from build123d import *

# Parameters (mm, degrees)
BOSS_EXTRUDE2_DEPTH = 6.35
CUT_EXTRUDE1_DEPTH  = 7.3500001
BOSS_EXTRUDE3_DEPTH = 6.35
SKETCH10_R          = 3.96875
CUT_EXTRUDE2_DEPTH  = 7.35
SKETCH11_R          = 4.5
CUT_EXTRUDE4_DEPTH  = 7.35
BOSS_EXTRUDE4_DEPTH = 6.35
SKETCH13_R          = 3.96875
CUT_EXTRUDE5_DEPTH  = 7.35
LPATTERN1_COUNT     = 2
LPATTERN1_PITCH     = 64
SKETCH14_R          = 2.54
CUT_EXTRUDE6_DEPTH  = 7.35
SKETCH15_R          = 3.96875
CUT_EXTRUDE7_DEPTH  = 7.35
SKETCH16_R          = 3.96875
CUT_EXTRUDE8_DEPTH  = 7.35
SKETCH19_R          = 3.96875
CUT_EXTRUDE11_DEPTH = 7.35
SKETCH21_R          = 2.54
CUT_EXTRUDE12_DEPTH = 7.35
SKETCH22_R          = 31.75
CUT_EXTRUDE13_DEPTH = 7.35
SKETCH23_R          = 5.807663874
SKETCH23_R_2        = 5.610358505
BOSS_EXTRUDE5_DEPTH = 6.35
SKETCH24_R          = 10.761293976
SKETCH24_R_2        = 16.881729782
SKETCH24_R_3        = 7.918988805
BOSS_EXTRUDE6_DEPTH = 6.35
CUT_EXTRUDE14_DEPTH = 7.35
FILLET1_R           = 3.175


with BuildPart() as part:
    # Sketch6 → Boss-Extrude2 (new body)
    with BuildSketch(Plane.XY):
        with BuildLine():
            Line((-68.006850091, -76.67090114), (-109.486767671, -48.656527855))
            Line((-109.486767671, -48.656527855), (-118.371760678, -61.812230963))
            Line((-118.371760678, -61.812230963), (18.447551645, -154.216158235))
            Line((18.447551645, -154.216158235), (135.729459338, 19.43912279))
            Line((135.729459338, 19.43912279), (-1.089852986, 111.843050063))
            Line((-1.089852986, 111.843050063), (-73.946795643, 3.966284577))
            Line((-73.946795643, 3.966284577), (-56.624438948, -7.732749433))
            ThreePointArc((-56.624438948, -7.732749433), (-43.058385537, 37.577891571), (0, 57.15))
            ThreePointArc((0, 57.15), (56.404848571, 31.095576642), (70.829334649, -29.338471048))
            add(Edge.make_bspline(
                [(70.829334649, -29.338471048), (70.811686062, -29.418295928), (70.776015112, -29.578104383), (70.713320217, -29.85478305), (70.619021771, -30.262929245), (70.501052001, -30.762086912), (70.364034474, -31.322191481), (70.199318515, -31.970958926), (70.000453855, -32.723919765), (69.795103485, -33.469783355), (69.582015398, -34.214296028), (69.361377803, -34.956693289), (69.133257682, -35.696762218), (68.838782679, -36.61892651), (68.470566207, -37.720710028), (68.019498024, -38.998776477), (67.474836154, -40.448808619), (66.901337925, -41.887676852), (66.299328392, -43.31485223), (65.669141732, -44.729810424), (65.011119088, -46.132040323), (64.325609411, -47.52103904), (63.612968547, -48.896314904), (62.87355937, -50.257385735), (62.107751613, -51.603779381), (61.315921169, -52.935034173), (60.49845004, -54.250698756), (59.655726138, -55.550331897), (58.571247582, -57.154294757), (57.220953058, -59.045283389), (55.576035723, -61.200397094), (53.604026134, -63.590264702), (51.54329346, -65.904053004), (49.39728314, -68.138962994), (47.169496434, -70.29235602), (44.863486103, -72.361752995), (42.482847363, -74.344831806), (40.031215607, -76.239428526), (36.882516177, -78.494556171), (32.976808929, -81.016011003), (28.250788286, -83.68089187), (21.41551215, -86.919136497), (14.30829026, -89.526654921), (6.996956895, -91.488176442), (-0.451922312, -92.797413176), (-6.61686174, -93.456358442), (-12.81195397, -93.702029749), (-19.009644204, -93.537285056), (-25.183124422, -92.966685286), (-31.306438312, -91.996382122), (-36.598524037, -90.804323442), (-41.072542301, -89.543185606), (-44.752319298, -88.33589156), (-47.664184976, -87.27761875), (-50.541347258, -86.128353728), (-53.381128552, -84.889612663), (-56.180924218, -83.562977818), (-58.593536599, -82.326710176), (-60.633378351, -81.214215821), (-62.313751085, -80.252471782), (-63.646071553, -79.462491566), (-64.966093336, -78.652178853), (-66.222359154, -77.854259082), (-67.143044791, -77.250601571), (-67.736251212, -76.85365602), (-68.006850091, -76.67090114)],
                knots=[0.071020771, 0.071020771, 0.071020771, 0.071020771, 0.071020771, 0.072848477, 0.074676184, 0.07650389, 0.078331597, 0.08198701, 0.085642423, 0.089297836, 0.092953249, 0.096608662, 0.100264075, 0.103919488, 0.107574901, 0.114885727, 0.122196554, 0.12950738, 0.136818214, 0.144129048, 0.151439882, 0.158750716, 0.166061558, 0.173372401, 0.180683243, 0.187994085, 0.195304924, 0.202615763, 0.209926602, 0.217237441, 0.231859103, 0.246480766, 0.261102426, 0.275724085, 0.290345754, 0.304967424, 0.319589099, 0.334210774, 0.348832457, 0.36345414, 0.392697464, 0.421940789, 0.451184112, 0.506140643, 0.535383973, 0.564627303, 0.593870641, 0.623113979, 0.652357319, 0.68160066, 0.710843985, 0.740087309, 0.754708984, 0.769330659, 0.783952333, 0.798574008, 0.813195669, 0.82781733, 0.842438991, 0.849749821, 0.857060652, 0.86437149, 0.871682327, 0.878993165, 0.885158103, 0.885158103, 0.885158103, 0.885158103, 0.885158103], degree=4))
        make_face()
    extrude(amount=BOSS_EXTRUDE2_DEPTH)

    # Sketch8 → Cut-Extrude1 (cut, through all)
    with BuildSketch(Plane.XY.offset(6.35)):
        Polygon((-71.011229489, -93.798205788), (-53.378672597, -90.381637707), (-42.854110111, -97.489632113), (-39.43754203, -115.122189004), align=None)
    extrude(amount=-CUT_EXTRUDE1_DEPTH, mode=Mode.SUBTRACT)

    # Sketch9 → Boss-Extrude3 (add, through all)
    with BuildSketch(Plane.XY.offset(6.35)):
        Polygon((-1.089852986, 111.843050063), (-109.486767671, -48.656527855), (27.332544652, -141.060455127), (135.729459338, 19.43912279), align=None)
    extrude(amount=-BOSS_EXTRUDE3_DEPTH)

    # Sketch10 → Cut-Extrude2 (cut, through all)
    with BuildSketch(Plane.XY.offset(6.35)):
        with Locations((4.996496209, -84.796642912)):
            Circle(SKETCH10_R)
        with Locations((40.816310536, -31.759477627)):
            Circle(SKETCH10_R)
        with Locations((76.636124864, 21.277687659)):
            Circle(SKETCH10_R)
        with Locations((-45.295165913, -45.214466102)):
            Circle(SKETCH10_R)
    extrude(amount=-CUT_EXTRUDE2_DEPTH, mode=Mode.SUBTRACT)

    # Sketch11 → Cut-Extrude4 (cut, through all)
    with BuildSketch(Plane.XY.offset(6.35)):
        Circle(SKETCH11_R)
    extrude(amount=-CUT_EXTRUDE4_DEPTH, mode=Mode.SUBTRACT)

    # Sketch12 → Boss-Extrude4 (add, through all)
    with BuildSketch(Plane.XY.offset(6.35)):
        Polygon((135.729459338, 19.43912279), (67.319803176, 65.641086427), (88.643786393, 97.214773886), (157.053442554, 51.01281025), align=None)
    extrude(amount=-BOSS_EXTRUDE4_DEPTH)

    # Sketch13 → Cut-Extrude5 (cut, through all)
    with BuildSketch(Plane.XY.offset(6.35)):
        with Locations((94.899221836, -29.671127724)):
            Circle(SKETCH13_R)
    cut_extrude5 = extrude(amount=-CUT_EXTRUDE5_DEPTH, mode=Mode.SUBTRACT)

    # LPattern1: Cut-Extrude5 ×2
    with Locations(*[Vector(-0.559684599, -0.828705708, 0) * (i * LPATTERN1_PITCH) for i in range(1, LPATTERN1_COUNT)]):
        add(cut_extrude5, mode=Mode.SUBTRACT)

    # Sketch14 → Cut-Extrude6 (cut, through all)
    with BuildSketch(Plane.XY.offset(6.35)):
        with Locations((71.72703343, -52.635713164)):
            Circle(SKETCH14_R)
        with Locations((35.907219102, -105.67287845)):
            Circle(SKETCH14_R)
        with Locations((115.740620068, 63.589229581)):
            Circle(SKETCH14_R)
    extrude(amount=-CUT_EXTRUDE6_DEPTH, mode=Mode.SUBTRACT)

    # Sketch15 → Cut-Extrude7 (cut, through all)
    with BuildSketch(Plane.XY.offset(6.35)):
        with Locations((-105.147343009, -59.249804902)):
            Circle(SKETCH15_R)
        with Locations((15.885125585, -140.991740566)):
            Circle(SKETCH15_R)
        with Locations((1.472573075, 98.618632394)):
            Circle(SKETCH15_R)
    extrude(amount=-CUT_EXTRUDE7_DEPTH, mode=Mode.SUBTRACT)

    # Sketch16 → Cut-Extrude8 (cut, through all)
    with BuildSketch(Plane.XY.offset(6.35)):
        with Locations((92.060354474, 79.582216994)):
            Circle(SKETCH16_R)
        with Locations((139.420885662, 47.596242169)):
            Circle(SKETCH16_R)
    extrude(amount=-CUT_EXTRUDE8_DEPTH, mode=Mode.SUBTRACT)

    # Sketch19 → Cut-Extrude11 (cut, through all)
    with BuildSketch(Plane.XY.offset(6.35)):
        with Locations((-65.680233685, -85.904783923)):
            Circle(SKETCH19_R)
    extrude(amount=-CUT_EXTRUDE11_DEPTH, mode=Mode.SUBTRACT)

    # Sketch21 → Cut-Extrude12 (cut, through all)
    with BuildSketch(Plane.XY.offset(6.35)):
        with Locations((-13.666272317, 70.530227577)):
            Circle(SKETCH21_R)
        with Locations((26.00698069, 78.217505758)):
            Circle(SKETCH21_R)
        with Locations((-86.729358658, -71.688795112)):
            Circle(SKETCH21_R)
        with Locations((-8.64928203, -120.590613931)):
            Circle(SKETCH21_R)
    extrude(amount=-CUT_EXTRUDE12_DEPTH, mode=Mode.SUBTRACT)

    # Sketch22 → Cut-Extrude13 (cut, through all)
    with BuildSketch(Plane.XY.offset(6.35)):
        Circle(SKETCH22_R)
    extrude(amount=-CUT_EXTRUDE13_DEPTH, mode=Mode.SUBTRACT)

    # Sketch23 → Boss-Extrude5 (add, through all)
    with BuildSketch(Plane.XY.offset(6.35)):
        with Locations((-65.680233685, -85.904783923)):
            Circle(SKETCH23_R)
        with Locations((-86.729358658, -71.688795112)):
            Circle(SKETCH23_R_2)
    extrude(amount=-BOSS_EXTRUDE5_DEPTH)

    # Sketch24 → Boss-Extrude6 (add, through all)
    with BuildSketch(Plane.XY.offset(6.35)):
        with Locations((-45.295165913, -45.214466102)):
            Circle(SKETCH24_R)
        with Locations((4.996496209, -84.796642912)):
            Circle(SKETCH24_R_2)
        with Locations((40.816310536, -31.759477627)):
            Circle(SKETCH24_R_3)
    extrude(amount=-BOSS_EXTRUDE6_DEPTH)

    # Sketch25 → Cut-Extrude14 (cut, through all)
    with BuildSketch(Plane.XY.offset(6.35)):
        Polygon((85.800588631, 93.004948891), (87.167215863, 85.951926135), (71.529628171, 62.797888664), (67.319803176, 65.641086427), align=None)
    extrude(amount=-CUT_EXTRUDE14_DEPTH, mode=Mode.SUBTRACT)

    # Fillet1
    fillet1_edges = [part.edges().sort_by_distance(p)[0] for p in [
        (-1.089852986, 111.843050063, 3.175),
        (18.447551645, -154.216158235, 3.175),
        (-118.371760678, -61.812230963, 3.175),
        (85.800588631, 93.004948891, 3.175),
        (87.167215863, 85.951926135, 3.175),
        (71.529628171, 62.797888664, 3.175),
        (-39.43754203, -115.122189004, 3.175),
        (-71.011229489, -93.798205788, 3.175),
        (-53.378672597, -90.381637707, 3.175),
        (-42.854110111, -97.489632113, 3.175),
        (157.053442554, 51.01281025, 3.175),
        (88.643786393, 97.214773886, 3.175),
    ]]
    fillet(fillet1_edges, radius=FILLET1_R)


solid = part.part
Build history of the part. All positions in model axes, mm. A direction names the side the tool comes from. Round coordinates to 2 decimals unless told otherwise and drop trailing zeros. Write each loop counter-clockwise with the first axis right and the second up, starting at its lowest first coordinate (ties: lowest second). Pieces come first, ordered by that corner, then holes. Notation, with made-up numbers: M 58.5,68.25 L 95.5,68.25 A19 ccw 95.5,82.25 Z; hole C 2,-6 d8. An arc over 180 degrees is marked long. Use CSV: the item, a comma, the result in double quotes.
1. Saw through at C-C (y = 57). Give the cut face in (x, z), plus the area to 3 significant figures.
Reply:
outline,"M -38.13,0 L 148.19,0 L 148.19,6.35 L -38.13,6.35 Z"
area,"1,180 mm²"
2. Tool access for faces 4 (the face through (72.67, 21.45, 3.22)), 5 (the face through (-48.17, -93.9, 3.22)): list every direction of +Z, -Z, +X, -X, +Y, -Y with a clear straight run to the whole face (end or side of a thin tool).
Reply:
face 4,"+Z, -Z"
face 5,"+Z, -Z, -Y"
3. Wall check: probe 1 along Y at (x, z) = (-10, 3.25); probe 2 along Y at (x, z) = (94, 5); probe 3 along Y at (x, z) = (-4, 0.5). Give the ranges that are in metal, low to high. Write a range as from..to.
Reply:
probe 1,"y = -135..-122.74, -118.44..-30.13, 30.13..98.65"
probe 2,"y = -42.35..-33.54, -25.81..76.12, 83.04..93.6"
probe 3,"y = -139.06..-31.5, 31.5..107.53"
4. Flat gauge pins, fed straight in: pin 1 (6.5 mm diameter, centred on x = 139.42, y = 47.6, fed in from +Z); pin 2 (1.5 mm diameter, centred on y = 68, z = 3.5, fed in from -X); pin 3 (2 mm diameter, centred on y = -12.5, z = 5, fed in from +X). Where does each tip first touch, or does it go through?
Reply:
pin 1,"passes through"
pin 2,"stops at x = -31.21"
pin 3,"stops at x = 114.83"
5. Saw through at B-B (z = 4.25). State how many separate pieces and enclosed holes the cut face has, plus the area to 3 significant figures.
Reply:
separate pieces,"1"
enclosed holes,"15"
area,"33,600 mm²"
6. Saw through at A-A (y = 0). Give the cut face in (x, z).
Reply:
outline,"M -76.63,0 L -31.75,0 L -31.75,6.35 L -76.63,6.35 Z; M 31.75,0 L 122.6,0 L 122.6,6.35 L 31.75,6.35 Z"
7. Two-plate mould, pull along Y, no slides. Class faces 1 (the face through (136.27, 45.18, 3.22)), 2 (the face through (-94.226, -78.119, 3.131)), 3 (the face through (122.41, 74.41, 3.22)): +Y half, -Y half, draft (parallel to the pull), parting line (faces both ways), or undercut.
Reply:
face 1,"undercut"
face 2,"-Y half"
face 3,"+Y half"
